```python
from build123d import *

# Parameters (mm, degrees)
SKETCH1_R           = 2.5
SKETCH1_W           = 4.3
SKETCH1_H           = 2.3
BOSS_EXTRUDE1_DEPTH = 10
SKETCH2_W           = 4
SKETCH2_H           = 59.39567842
CUT_EXTRUDE1_DEPTH  = 3
FILLET3_R           = 5
CHAMFER2_SIZE       = 4
SKETCH3_R           = 2.5
CUT_EXTRUDE2_DEPTH  = 10


with BuildPart() as part:
    # Sketch1 → Boss-Extrude1 (new body)
    with BuildSketch(Plane(origin=(0, 0, 0), x_dir=(1, 0, 0), z_dir=(0, 1, 0))):
        Polygon((0, -25), (0, 25), (15, 25), (15, -8), (20, -18), (32, -18), (35, -18), (120, -18), (120, -33), (4, -33), align=None)
        with Locations(Location((5, 20, 0), (0, 0, 270))):
            Circle(SKETCH1_R, mode=Mode.SUBTRACT)
        with Locations(Location((5, -20, 0), (0, 0, 270))):
            Circle(SKETCH1_R, mode=Mode.SUBTRACT)
        with Locations((27.51, -20.72)):
            Rectangle(SKETCH1_W, SKETCH1_H, mode=Mode.SUBTRACT)
    extrude(amount=BOSS_EXTRUDE1_DEPTH)

    # Sketch2 → Cut-Extrude1 (cut)
    with BuildSketch(Plane.XZ):
        with Locations((12, 4.69783921)):
            Rectangle(SKETCH2_W, SKETCH2_H)
    extrude(amount=-CUT_EXTRUDE1_DEPTH, mode=Mode.SUBTRACT)

    # Fillet3
    fillet3_edges = [part.edges().sort_by_distance(p)[0] for p in [
        (120, 5, 33),
        (120, 5, 18),
        (0, 5, -25),
        (15, 5, -25),
    ]]
    fillet(fillet3_edges, radius=FILLET3_R)

    # Chamfer2
    # the kernel refuses this chamfer: 4 mm, written as the material it takes off along each edge
    with BuildSketch(Plane(origin=(20.286731952, 0, 33), x_dir=(0, -0.027495876610586365, -0.9996219169112968), z_dir=(-1, 0, 0))) as chamfer2_piece_1:
        Polygon((CHAMFER2_SIZE * 0.999621916911, -CHAMFER2_SIZE * 0.0274958766106), (-CHAMFER2_SIZE * 0.0274958766106, -CHAMFER2_SIZE * 0.999621916911), (0, 0), align=None)
    extrude(amount=26.573463904, mode=Mode.SUBTRACT)
    with BuildSketch(Plane(origin=(115, 0, 33), x_dir=(0, 0.9996219169112968, 0.02749587661058563), z_dir=(-1, 0, 0))) as chamfer2_piece_2:
        Polygon((CHAMFER2_SIZE * 0.999621916911, CHAMFER2_SIZE * 0.0274958766106), (-CHAMFER2_SIZE * 0.0274958766106, CHAMFER2_SIZE * 0.999621916911), (0, 0), align=None)
    extrude(amount=111.286731952, mode=Mode.SUBTRACT)
    with BuildSketch(Plane(origin=(120, 0, 23), x_dir=(0.02749587661058563, 0.9996219169112968, 0), z_dir=(0, 0, 1))) as chamfer2_piece_3:
        Polygon((CHAMFER2_SIZE * 0.999621916911, CHAMFER2_SIZE * 0.0274958766106), (-CHAMFER2_SIZE * 0.0274958766106, CHAMFER2_SIZE * 0.999621916911), (0, 0), align=None)
    extrude(amount=5, mode=Mode.SUBTRACT)
    with BuildSketch(Plane(origin=(115, 0, 18), x_dir=(0, 0.999621916911297, -0.02749587661058045), z_dir=(-1, 0, 0))) as chamfer2_piece_4_section:
        Polygon((CHAMFER2_SIZE * 0.999621916911, -CHAMFER2_SIZE * 0.0274958766106), (-CHAMFER2_SIZE * 0.0274958766106, -CHAMFER2_SIZE * 0.999621916911), (0, 0), align=None)
    chamfer2_piece_4 = extrude(amount=105.286731952, mode=Mode.PRIVATE)
    chamfer2_piece_4 = split(chamfer2_piece_4, bisect_by=Plane(origin=(30.091205291, 1.322053336, 38.182410583), z_dir=(0.8944271909999159, 0, -0.4472135954999581)), keep=Keep.TOP, mode=Mode.PRIVATE)
    add(chamfer2_piece_4, mode=Mode.SUBTRACT)
    with BuildSketch(Plane(origin=(115, 0, 23), x_dir=(0, 0, -1), z_dir=(-1, 0, 0))) as chamfer2_piece_5:
        Polygon((5, -CHAMFER2_SIZE), (5 - CHAMFER2_SIZE, 0), (5, 0), align=None)
    revolve(axis=Axis((115, 0, 23), (0, -1, 0)), revolution_arc=90, mode=Mode.SUBTRACT)
    with BuildSketch(Plane(origin=(115, 0, 28), x_dir=(0, 0, 1), z_dir=(-1, 0, 0))) as chamfer2_piece_6:
        Polygon((5, CHAMFER2_SIZE), (5 - CHAMFER2_SIZE, 0), (5, 0), align=None)
    revolve(axis=Axis((115, 0, 28), (0, 1, 0)), revolution_arc=90, mode=Mode.SUBTRACT)

    # Sketch3 → Cut-Extrude2 (cut)
    with BuildSketch(Plane.XZ):
        with Locations(Location((27.5, 27, 0), (0, 0, 270))):
            Circle(SKETCH3_R)
    extrude(amount=-CUT_EXTRUDE2_DEPTH, mode=Mode.SUBTRACT)


solid = part.part
```
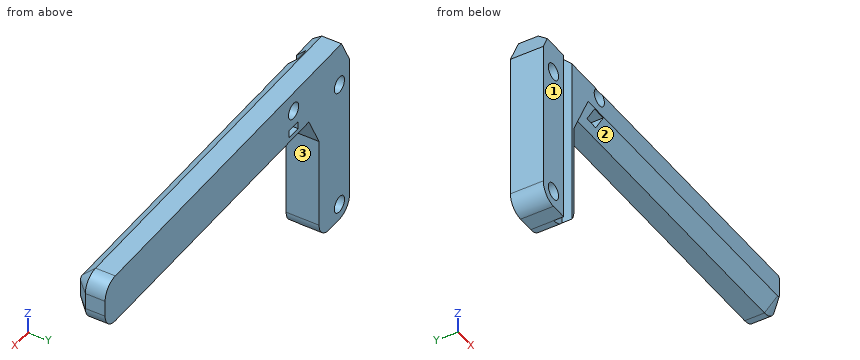
Can you work these out from the model? Positions are in its coordinate system, mm. Face numbers are marked on the shaded views. A direction names the side the tool comes from. Round coordinates to 2 decimals unless told otherwise and drop trailing zeros. Loops run counter-clockwise (first coordinate to the right, second up) from the corner with the lowest first, then second, coordinate; pieces in that order, holes last. Notation, with made-up numbers: M 52.5,-35 L 71.5,-35 A7 cw 71.5,-30 Z; hole C -25.75,-39 d3. An arc over 180 degrees is marked long. Answer in a Markdown table with one row per item.
1. On a 3-axis mill with a long thin cutter (end or side, diameter ignored), from which of +Z, -Z, +X, -X, +Y, -Y can I reach the whole of each face in a straight line? I mean the marked faces 1, 2 and 3. Say none if no direction works.
Established:
| item | result |
|---|---|
| face 1 | +Z, -Z, +X, -X, -Y |
| face 2 | -Z, +X, -Y |
| face 3 | -Z, +X, +Y, -Y |
2. If we section it at B-B, the plane z = -12.5: Please give me the cut outline in (x, y).
Established:
| item | result |
|---|---|
| outline | M 0,0 L 10,0 L 10,3 L 14,3 L 14,0 L 15,0 L 15,10 L 0,10 Z |
3. I'm going to push flat-ended pins straight in: pin 1 Ø3 at (y, z) = (6.5, -4.5) entering from +X; pin 2 Ø1.2 at (y, z) = (5.5, 20) entering from +X; pin 3 Ø5 at (x, y) = (71, 7) entering from -Z. Where does each tip first touch, or does it pass through?
Established:
| item | result |
|---|---|
| pin 1 | x = 15 |
| pin 2 | x = 119.39 |
| pin 3 | z = 18 |
4. If we section it at A-A, the plane x = 27.5: Please give me the cut outline in (y, z).
Established:
| item | result |
|---|---|
| outline | M 0,22 L 0.13,21.87 L 10,21.87 L 10,24.5 L 0,24.5 Z; M 0.5,29.5 L 10,29.5 L 10,33 L 4,33 Z; M 2.43,19.57 L 4,18 L 10,18 L 10,19.57 Z |
5. Please list where these lines run through material, in increasing order: line 1 (Z direction, x = 27.5, y = 7.25); line 2 (Z direction, x = 6, y = 3.5); line 3 (Z direction, x = 54.5, y = 7.75). Write a range as from..to.
Established:
| item | result |
|---|---|
| line 1 | 18..19.57, 21.87..24.5, 29.5..33 |
| line 2 | -25..-22.29, -17.71..17.71, 22.29..32.5 |
| line 3 | 18..33 |
6. If we section it at C-C, the plane x = 91.5: Please give me the cut outline in (y, z).
Established:
| item | result |
|---|---|
| outline | M 0,22 L 4,18 L 10,18 L 10,33 L 4,33 L 0,29 Z |
